from build123d import *

# Parameters (mm, degrees)
SKETCH047_W             = 19.5
SKETCH047_H             = 27
PAD028_DEPTH            = 15
SKETCH048_W             = 22.5
SKETCH048_H             = 30
PAD027_DEPTH            = 2
POCKET019_DEPTH         = 12.5
SKETCH046_R             = 3.5
POCKET018_DEPTH         = 50
BODY015_ROLL_ANGLE      = 180
BODY015_PLACEMENT_ANGLE = -90


with BuildPart() as part:
    # Sketch047 → Pad028 (new body)
    with BuildSketch(Plane.XY):
        with Locations((9.75, 13.5)):
            Rectangle(SKETCH047_W, SKETCH047_H)
    extrude(amount=PAD028_DEPTH)

    # Sketch048 → Pad027 (join)
    with BuildSketch(Plane.XY.offset(2)):
        with Locations((8.25, 15)):
            Rectangle(SKETCH048_W, SKETCH048_H)
    extrude(amount=PAD027_DEPTH)

    # Sketch045 → Pocket019 (cut)
    with BuildSketch(Plane.XY):
        with BuildLine():
            ThreePointArc((18.75, 15), (9.749994, 24), (0.75, 14.999989))
            Line((0.75, 14.999989), (0.75, 0))
            Line((0.75, 0), (18.75, 0))
            Line((18.75, 0), (18.75, 15))
        make_face()
    extrude(amount=POCKET019_DEPTH, mode=Mode.SUBTRACT)

    # Sketch046 → Pocket018 (cut, symmetric)
    with BuildSketch(Plane.XY):
        with Locations((9.75, 15)):
            Circle(SKETCH046_R)
    extrude(amount=POCKET018_DEPTH, both=True, mode=Mode.SUBTRACT)


with BuildPart() as part_1:
    # Body015 roll: moved
    add(part.part.rotate(Axis((0, 0, 0), (1, 0, 0)), BODY015_ROLL_ANGLE))


with BuildPart() as part_2:
    # Body015 placement: moved
    add(part_1.part.moved(Location((65.5, 90.092583, -0.881905))).rotate(Axis((65.5, 90.092583, -0.881905), (0, 0, 1)), BODY015_PLACEMENT_ANGLE))


solid = part_2.part
The listing builds one solid part. Answer for the finished solid, in the listing's coordinates (mm). A direction names the side the tool comes from. Give positions to 0.01 mm unless a question says otherwise; leave off trailing zeros. Loops run counter-clockwise (first coordinate to the right, second up) from the corner with the lowest first, then second, coordinate; pieces in that order, holes last. Notation, with made-up numbers: (-32.75, -36) - (2.25, -36) arc R12 ccw to (2.25, -30) - close; hole circle Ø9 at (-34, -27.75). An arc over 180 degrees is marked (long way). Write each question's results on one line, items separated by ' | '.
1. Flat-ended cylindrical pins translate along their axes: P1, Ø5, axis at y = 75.5, z = -12, coming from the +X side; P2, Ø9, axis at x = 55, y = 83.5, coming from the +Z side; P3, Ø3, axis at x = 56, z = -12, coming from the +Y side; P4, Ø4, axis at y = 81, z = -9.5, coming from the +X side. Find the tip coordinate at first contact, or state that the pin passes through.
Resolved:
P1: stops at x = 65.5 | P2: stops at z = -13.38 | P3: stops at y = 90.09 | P4: stops at x = 41.9
2. Consider probe 1 along Y at (x, z) = (50.5, -15.1); probe 2 along Y at (x, z) = (51, -6); probe 3 along Z at (x, y) = (45.75, 81.75). Determine where each line is inside the solid, lowest interval first. Write a range as from..to.
Resolved:
probe 1: y = 70.59..76.84, 83.84..90.09 | probe 2: y = 70.59..71.34, 89.34..90.09 | probe 3: z = -15.88..-13.38
3. For a pull along Y with two mould halves and no side action, classify faces 5 (the face through (51, 93.093, -4)), 6 (the face through (38.5, 80, -10)), 7 (the face through (58, 89.343, -7)) as +Y half, -Y half, draft (parallel to the pull), parting line (faces both ways), or undercut.
Resolved:
face 5: +Y half | face 6: draft | face 7: undercut
4. Find section D-D, the plane y = 78. Write down the section's boundary in (x, z).
Resolved:
outline: (35.5, -4.88) - (38.5, -4.88) - (38.5, -15.88) - (47.9, -15.88) - (47.9, -13.38) - (41.81, -13.38) - (41.81, -0.88) - (38.5, -0.88) - (38.5, -2.88) - (35.5, -2.88) - close; (53.1, -15.88) - (65.5, -15.88) - (65.5, -13.38) - (53.1, -13.38) - close
5. Find section C-C, the plane x = 51.5. Write down the section's boundary in (y, z).
Resolved:
outline: (70.59, -15.88) - (76.99, -15.88) - (76.99, -13.38) - (71.34, -13.38) - (71.34, -0.88) - (70.59, -0.88) - close; (83.7, -15.88) - (90.09, -15.88) - (90.09, -4.88) - (93.09, -4.88) - (93.09, -2.88) - (90.09, -2.88) - (90.09, -0.88) - (89.34, -0.88) - (89.34, -13.38) - (83.7, -13.38) - close
6. Find section B-B, the plane z = -13.75. Write down the section's boundary in (x, y).
Resolved:
outline: (38.5, 70.59) - (65.5, 70.59) - (65.5, 90.09) - (38.5, 90.09) - close; hole circle Ø7 at (50.5, 80.34)
7. Find section A-A, the plane x = 40.75. Write down the section's boundary in (y, z), then the cut area to 4 significant figures.
Resolved:
outline: (70.59, -15.88) - (90.09, -15.88) - (90.09, -4.88) - (93.09, -4.88) - (93.09, -2.88) - (90.09, -2.88) - (90.09, -0.88) - (70.59, -0.88) - close | area: 298.5 mm^2
8. Which of the six approach directions +Z, -Z, +X, -X, +Y, -Y give full straight-line access (tool end or side, diameter ignored) to faces 1 (the face through (52, 90.093, -2)), 2 (the face through (38.5, 80, -2)), 3 (the face through (52, 90.093, -10)), 4 (the face through (58, 71.343, -7))?
Resolved:
face 1: +Z, +X, -X, +Y | face 2: +Z, -X, +Y, -Y | face 3: -Z, +X, -X, +Y | face 4: +Z, +X
